Geometry check sheet. Reference: the model listing, model coordinates, mm. Coordinates: 2 decimals unless noted, no trailing zeros. Loops run counter-clockwise (first coordinate to the right, second up) from the corner with the lowest first, then second, coordinate; pieces in that order, holes last.
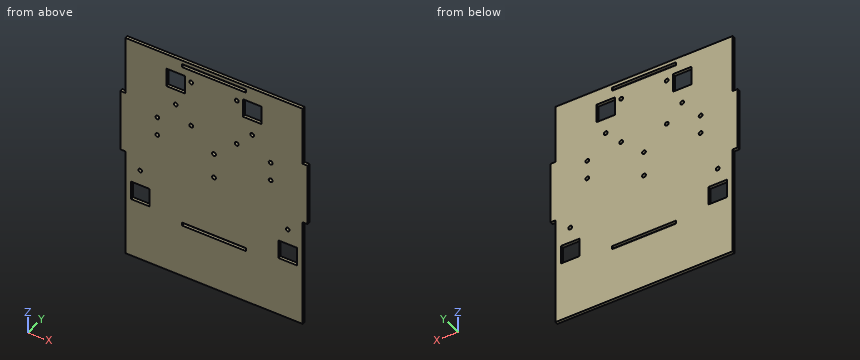
from build123d import *

# Parameters (mm, degrees)
SKETCH1_R           = 1.55
SKETCH1_W           = 15
SKETCH1_H           = 15
SKETCH1_W_2         = 52
SKETCH1_H_2         = 2.6
BOSS_EXTRUDE1_DEPTH = 2.5
SKETCH2_W           = 144
SKETCH2_H           = 40
BOSS_EXTRUDE2_DEPTH = 2.5


with BuildPart() as part:
    # Sketch1 → Boss-Extrude1 (new body)
    with BuildSketch(Plane(origin=(0, 0, 0), x_dir=(1, 0, 0), z_dir=(0, 1, 0))):
        Polygon((-72, -25), (-76, -25), (-76, 25), (-72, 25), (-72, 72.1), (72, 72.1), (72, 25), (76, 25), (76, -25), (72, -25), (72, -72.1), (-72, -72.1), align=None)
        with Locations((-18.5, -56.5)):
            Circle(SKETCH1_R, mode=Mode.SUBTRACT)
        with Locations((-18.5, -19.5)):
            Circle(SKETCH1_R, mode=Mode.SUBTRACT)
        with Locations((18.5, -19.5)):
            Circle(SKETCH1_R, mode=Mode.SUBTRACT)
        with Locations((18.5, -56.5)):
            Circle(SKETCH1_R, mode=Mode.SUBTRACT)
        with Locations((0, -3)):
            Circle(SKETCH1_R, mode=Mode.SUBTRACT)
        with Locations((0, 17)):
            Circle(SKETCH1_R, mode=Mode.SUBTRACT)
        with Locations((-59.898406921, 36.347928242)):
            Circle(SKETCH1_R, mode=Mode.SUBTRACT)
        with Locations((59.898406921, 36.347928242)):
            Circle(SKETCH1_R, mode=Mode.SUBTRACT)
        with Locations((31.018932052, -32.377895768)):
            Circle(SKETCH1_R, mode=Mode.SUBTRACT)
        with Locations((-31.018932052, -32.377895768)):
            Circle(SKETCH1_R, mode=Mode.SUBTRACT)
        with Locations((-46, -15)):
            Circle(SKETCH1_R, mode=Mode.SUBTRACT)
        with Locations((-46, 0)):
            Circle(SKETCH1_R, mode=Mode.SUBTRACT)
        with Locations((46, -15)):
            Circle(SKETCH1_R, mode=Mode.SUBTRACT)
        with Locations((46, 0)):
            Circle(SKETCH1_R, mode=Mode.SUBTRACT)
        with Locations((59.898406921, 56.347928242)):
            Rectangle(SKETCH1_W, SKETCH1_H, mode=Mode.SUBTRACT)
        with Locations((-59.898406921, 56.347928242)):
            Rectangle(SKETCH1_W, SKETCH1_H, mode=Mode.SUBTRACT)
        with Locations((31.018932052, -52.377895768)):
            Rectangle(SKETCH1_W, SKETCH1_H, mode=Mode.SUBTRACT)
        with Locations((-31.018932052, -52.377895768)):
            Rectangle(SKETCH1_W, SKETCH1_H, mode=Mode.SUBTRACT)
        with Locations((0, -67.8)):
            Rectangle(SKETCH1_W_2, SKETCH1_H_2, mode=Mode.SUBTRACT)
        with Locations((0, 67.8)):
            Rectangle(SKETCH1_W_2, SKETCH1_H_2, mode=Mode.SUBTRACT)
    extrude(amount=BOSS_EXTRUDE1_DEPTH)

    # Sketch2 → Boss-Extrude2 (add)
    with BuildSketch(Plane(origin=(0, 2.5, 0), x_dir=(1, 0, 0), z_dir=(0, 1, 0))):
        with Locations((0, 92.1)):
            Rectangle(SKETCH2_W, SKETCH2_H)
    extrude(amount=-BOSS_EXTRUDE2_DEPTH)


solid = part.part
(1) Scan lines: L1, parallel to Z at x = 0, y = 0.8; L2, parallel to X at y = 0.8, z = 0; L3, parallel to Z at x = -46, y = 1.85. Record each from-to range of solid material in increasing order.
Findings:
L1: z = -112.1 to -69.1, -66.5 to -18.55, -15.45 to 1.45, 4.55 to 66.5, 69.1 to 72.1
L2: x = -76 to -47.55, -44.45 to 44.45, 47.55 to 76
L3: z = -112.1 to -1.55, 1.55 to 13.45, 16.55 to 72.1
(2) Gauge pin test, flat end, axial feed: pin 1 Ø0.8 at (y, z) = (1.5, 55.5) entering from -X. Record the tip position at first contact, or that the pin passes through.
Findings:
pin 1: stops at x = -72
(3) Sectioned sample at A-A on z = 48. Record the cut outline in (x, y), and give its area (3 significant figures).
Findings:
outline: (-72, 0) - (-38.52, 0) - (-38.52, 2.5) - (-72, 2.5) - close; (-23.52, 0) - (23.52, 0) - (23.52, 2.5) - (-23.52, 2.5) - close; (38.52, 0) - (72, 0) - (72, 2.5) - (38.52, 2.5) - close
area: 285 mm2
(4) Sectioned sample at B-B on z = -83.5. Record the cut outline in (x, y).
Findings:
outline: (-72, 0) - (72, 0) - (72, 2.5) - (-72, 2.5) - close
(5) Sectioned sample at C-C on y = 0.5. State how many separate pieces and enclosed holes the cut face has, and give its area (3 significant figures).
Findings:
separate pieces: 1
enclosed holes: 20
area: 25,600 mm2
